Input: part model. Units: mm. Frame: model coordinates. A direction names the side the tool comes from. Coordinates: 2 decimals unless noted, no trailing zeros. Write each loop counter-clockwise with the first axis right and the second up, starting at its lowest first coordinate (ties: lowest second). Pieces come first, ordered by that corner, then holes. Notation, with made-up numbers: M -30,-21 L -9,-21 A23 cw -9,-7 Z; hole C 21,37 d11. An arc over 180 degrees is marked long. Write each question's results on one line, items separated by ' | '. Start each with the question number.
1. Ray query, probe 1 along X at (y, z) = (-0.75, 62); probe 2 along Z at (x, y) = (90.5, -0.2); probe 3 along Z at (x, y) = (55, -0.25). Return the intervals inside material, ascending.
2. Section query A-A, the plane y = -0.9. Output: boundary loops of the cut face in (x, z).
3. Pull-direction query (X, two-part tool) for faces 3 (the cylindrical face through (50.28, -0.64, 93.09)), 4 (the cylindrical face through (6.014, 0.21, 124.297)), 5 (the cylindrical face through (60, -0.6, 18.2)), 6 (the flat face through (65, -1.3, 106)); classes: +X half, -X half, draft (parallel to the pull), parting line (faces both ways), or undercut.
4. Section query D-D, the plane z = 106. Output: boundary loops of the cut face in (x, y).
5. Section query B-B, the plane z = 74. Output: boundary loops of the cut face in (x, y), and give its area (3 significant figures).
6. Section query C-C, the plane x = 69.9. Output: boundary loops of the cut face in (y, z).
7. First-contact query: pin 1 (4 mm diameter, centred on x = 24.5, z = 53, fed in from -Y); pin 2 (0.6 mm diameter, centred on y = -1, z = 36.5, fed in from -X); pin 3 (1 mm diameter, centred on y = 0.5, z = 113, fed in from +X). Flat tips, straight axial feed; report the tip coordinate or a pass-through.
8. Set-up query: faces 1 (the cylindrical face through (124.297, 0.21, 123.986)), 2 (the cylindrical face through (13.01, -0.25, 12.85)). Return all of +Z, -Z, +X, -X, +Y, -Y with unobstructed straight access to the full face (end or side cutting, diameter ignored); none if empty.
```python
from build123d import *

# Parameters (mm, degrees)
F1_DEPTH = 0.9
F2_DEPTH = 0.5
F3_DEPTH = 1.3


with BuildPart() as f1:
    # F0 (on Front) → F1 (new body)
    with BuildSketch(Plane.XZ):
        with BuildLine():
            ThreePointArc((0, 20), (5.857864, 5.857864), (20, 0))
            Line((20, 0), (65, 0))
            Line((65, 0), (110, 0))
            ThreePointArc((110, 0), (124.142136, 5.857864), (130, 20))
            Line((130, 20), (130, 110))
            ThreePointArc((130, 110), (124.142136, 124.142136), (110, 130))
            Line((110, 130), (65, 130))
            Line((65, 130), (20, 130))
            ThreePointArc((20, 130), (5.857864, 124.142136), (0, 110))
            Line((0, 110), (0, 20))
        make_face()
        with BuildLine():
            Line((65, 120), (110, 120))
            ThreePointArc((110, 120), (117.071068, 117.071068), (120, 110))
            Line((120, 110), (120, 20))
            ThreePointArc((120, 20), (117.071068, 12.928932), (110, 10))
            Line((110, 10), (65, 10))
            Line((65, 10), (20, 10))
            ThreePointArc((20, 10), (12.928932, 12.928932), (10, 20))
            Line((10, 20), (10, 110))
            ThreePointArc((10, 110), (12.928932, 117.071068), (20, 120))
            Line((20, 120), (65, 120))
        make_face(mode=Mode.SUBTRACT)
        with BuildLine():
            ThreePointArc((120, 110), (117.071068, 117.071068), (110, 120))
            Line((110, 120), (65, 120))
            Line((65, 120), (20, 120))
            ThreePointArc((20, 120), (12.928932, 117.071068), (10, 110))
            Line((10, 110), (10, 20))
            ThreePointArc((10, 20), (12.928932, 12.928932), (20, 10))
            Line((20, 10), (65, 10))
            Line((65, 10), (110, 10))
            ThreePointArc((110, 10), (117.071068, 12.928932), (120, 20))
            Line((120, 20), (120, 110))
        make_face()
        with BuildLine():
            ThreePointArc((47.212271, 85.792594), (50.201951, 93.01032), (57.419677, 96))
            Line((57.419677, 96), (65, 96))
            Line((65, 96), (72.580323, 96))
            ThreePointArc((72.580323, 96), (79.798049, 93.01032), (82.787729, 85.792594))
            Line((82.787729, 85.792594), (82.787729, 60.792594))
            ThreePointArc((82.787729, 60.792594), (79.493864, 57.498729), (76.2, 60.792594))
            Line((76.2, 60.792594), (76.2, 81.5))
            ThreePointArc((76.2, 81.5), (75.2, 82.5), (74.2, 81.5))
            Line((74.2, 81.5), (74.2, 22.5))
            ThreePointArc((74.2, 22.5), (69.9, 18.2), (65.6, 22.5))
            Line((65.6, 22.5), (65.6, 54.5))
            ThreePointArc((65.6, 54.5), (65.424264, 54.924264), (65, 55.1))
            ThreePointArc((65, 55.1), (64.575736, 54.924264), (64.4, 54.5))
            Line((64.4, 54.5), (64.4, 22.5))
            ThreePointArc((64.4, 22.5), (60.1, 18.2), (55.8, 22.5))
            Line((55.8, 22.5), (55.8, 81.5))
            ThreePointArc((55.8, 81.5), (54.8, 82.5), (53.8, 81.5))
            Line((53.8, 81.5), (53.8, 60.792594))
            ThreePointArc((53.8, 60.792594), (50.506136, 57.498729), (47.212271, 60.792594))
            Line((47.212271, 60.792594), (47.212271, 85.792594))
        make_face(mode=Mode.SUBTRACT)
        with BuildLine():
            ThreePointArc((65, 98.5), (57.5, 106), (65, 113.5))
            ThreePointArc((65, 113.5), (72.5, 106), (65, 98.5))
        make_face(mode=Mode.SUBTRACT)
        with BuildLine():
            Line((65, 96), (57.419677, 96))
            ThreePointArc((57.419677, 96), (50.201951, 93.01032), (47.212271, 85.792594))
            Line((47.212271, 85.792594), (47.212271, 60.792594))
            ThreePointArc((47.212271, 60.792594), (50.506136, 57.498729), (53.8, 60.792594))
            Line((53.8, 60.792594), (53.8, 81.5))
            ThreePointArc((53.8, 81.5), (54.8, 82.5), (55.8, 81.5))
            Line((55.8, 81.5), (55.8, 22.5))
            ThreePointArc((55.8, 22.5), (60.1, 18.2), (64.4, 22.5))
            Line((64.4, 22.5), (64.4, 54.5))
            ThreePointArc((64.4, 54.5), (64.575736, 54.924264), (65, 55.1))
            ThreePointArc((65, 55.1), (65.424264, 54.924264), (65.6, 54.5))
            Line((65.6, 54.5), (65.6, 22.5))
            ThreePointArc((65.6, 22.5), (69.9, 18.2), (74.2, 22.5))
            Line((74.2, 22.5), (74.2, 81.5))
            ThreePointArc((74.2, 81.5), (75.2, 82.5), (76.2, 81.5))
            Line((76.2, 81.5), (76.2, 60.792594))
            ThreePointArc((76.2, 60.792594), (79.493864, 57.498729), (82.787729, 60.792594))
            Line((82.787729, 60.792594), (82.787729, 85.792594))
            ThreePointArc((82.787729, 85.792594), (79.798049, 93.01032), (72.580323, 96))
            Line((72.580323, 96), (65, 96))
        make_face()
        with BuildLine():
            ThreePointArc((65, 98.5), (72.5, 106), (65, 113.5))
            ThreePointArc((65, 113.5), (57.5, 106), (65, 98.5))
        make_face()
    extrude(amount=-F1_DEPTH)

    # F0 (on Front) → F2 (join)
    with BuildSketch(Plane.XZ):
        with BuildLine():
            ThreePointArc((0, 20), (5.857864, 5.857864), (20, 0))
            Line((20, 0), (65, 0))
            Line((65, 0), (110, 0))
            ThreePointArc((110, 0), (124.142136, 5.857864), (130, 20))
            Line((130, 20), (130, 110))
            ThreePointArc((130, 110), (124.142136, 124.142136), (110, 130))
            Line((110, 130), (65, 130))
            Line((65, 130), (20, 130))
            ThreePointArc((20, 130), (5.857864, 124.142136), (0, 110))
            Line((0, 110), (0, 20))
        make_face()
        with BuildLine():
            Line((65, 120), (110, 120))
            ThreePointArc((110, 120), (117.071068, 117.071068), (120, 110))
            Line((120, 110), (120, 20))
            ThreePointArc((120, 20), (117.071068, 12.928932), (110, 10))
            Line((110, 10), (65, 10))
            Line((65, 10), (20, 10))
            ThreePointArc((20, 10), (12.928932, 12.928932), (10, 20))
            Line((10, 20), (10, 110))
            ThreePointArc((10, 110), (12.928932, 117.071068), (20, 120))
            Line((20, 120), (65, 120))
        make_face(mode=Mode.SUBTRACT)
    extrude(amount=F2_DEPTH)

    # F0 (on Front) → F3 (join)
    with BuildSketch(Plane.XZ):
        with BuildLine():
            ThreePointArc((65, 98.5), (72.5, 106), (65, 113.5))
            ThreePointArc((65, 113.5), (57.5, 106), (65, 98.5))
        make_face()
        with BuildLine():
            Line((65, 96), (57.419677, 96))
            ThreePointArc((57.419677, 96), (50.201951, 93.01032), (47.212271, 85.792594))
            Line((47.212271, 85.792594), (47.212271, 60.792594))
            ThreePointArc((47.212271, 60.792594), (50.506136, 57.498729), (53.8, 60.792594))
            Line((53.8, 60.792594), (53.8, 81.5))
            ThreePointArc((53.8, 81.5), (54.8, 82.5), (55.8, 81.5))
            Line((55.8, 81.5), (55.8, 22.5))
            ThreePointArc((55.8, 22.5), (60.1, 18.2), (64.4, 22.5))
            Line((64.4, 22.5), (64.4, 54.5))
            ThreePointArc((64.4, 54.5), (64.575736, 54.924264), (65, 55.1))
            ThreePointArc((65, 55.1), (65.424264, 54.924264), (65.6, 54.5))
            Line((65.6, 54.5), (65.6, 22.5))
            ThreePointArc((65.6, 22.5), (69.9, 18.2), (74.2, 22.5))
            Line((74.2, 22.5), (74.2, 81.5))
            ThreePointArc((74.2, 81.5), (75.2, 82.5), (76.2, 81.5))
            Line((76.2, 81.5), (76.2, 60.792594))
            ThreePointArc((76.2, 60.792594), (79.493864, 57.498729), (82.787729, 60.792594))
            Line((82.787729, 60.792594), (82.787729, 85.792594))
            ThreePointArc((82.787729, 85.792594), (79.798049, 93.01032), (72.580323, 96))
            Line((72.580323, 96), (65, 96))
        make_face()
    extrude(amount=F3_DEPTH)


solid = f1.part
```
Answer:
1) probe 1: 47.21 to 53.8, 55.8 to 74.2, 76.2 to 82.79 | probe 2: 0 to 10, 120 to 130 | probe 3: 0 to 10, 82.48 to 95.71, 120 to 130
2) outline: M 47.21,60.79 A3.29 ccw 53.8,60.79 L 53.8,81.5 A1 cw 55.8,81.5 L 55.8,22.5 A4.3 ccw 64.4,22.5 L 64.4,54.5 A0.6 cw 65.6,54.5 L 65.6,22.5 A4.3 ccw 74.2,22.5 L 74.2,81.5 A1 cw 76.2,81.5 L 76.2,60.79 A3.29 ccw 82.79,60.79 L 82.79,85.79 A10.21 ccw 72.58,96 L 57.42,96 A10.21 ccw 47.21,85.79 Z; C 65,106 d15
3) face 3: undercut | face 4: -X half | face 5: undercut | face 6: draft
4) outline: M 0,-0.5 L 10,-0.5 L 10,0 L 57.5,0 L 57.5,-1.3 L 72.5,-1.3 L 72.5,0 L 120,0 L 120,-0.5 L 130,-0.5 L 130,0.9 L 0,0.9 Z
5) outline: M 0,-0.5 L 10,-0.5 L 10,0 L 47.21,0 L 47.21,-1.3 L 53.8,-1.3 L 53.8,0 L 55.8,0 L 55.8,-1.3 L 74.2,-1.3 L 74.2,0 L 76.2,0 L 76.2,-1.3 L 82.79,-1.3 L 82.79,0 L 120,0 L 120,-0.5 L 130,-0.5 L 130,0.9 L 0,0.9 Z | area: 168 mm^2
6) outline: M -1.3,18.2 L 0,18.2 L 0,10 L -0.5,10 L -0.5,0 L 0.9,0 L 0.9,130 L -0.5,130 L -0.5,120 L 0,120 L 0,111.68 L -1.3,111.68 L -1.3,100.32 L 0,100.32 L 0,96 L -1.3,96 Z
7) pin 1: y = 0 | pin 2: x = 55.8 | pin 3: x = 129.84
8) face 1: +Z, +X, +Y, -Y | face 2: -Y
